Verification items for the finished model (mm, model axes). Give positions to 0.01 mm unless a question says otherwise; leave off trailing zeros. Loops run counter-clockwise (first coordinate to the right, second up) from the corner with the lowest first, then second, coordinate; pieces in that order, holes last. Notation, with made-up numbers: (33, -39) -> (78, -39) arc R12 cw to (78, -28) -> close; hole circle Ø9 at (-40, 40.5). An arc over 180 degrees is marked (long way). Answer in a Markdown table with one row per item. Add a question column.
Q1. Section check B-B on z = 18. Enter the section's corners in (x, y).
Q2. Section check C-C on x = -34.5. Enter the section's corners in (y, z).
Q3. Section check D-D on y = 0.95. Give the number of separate pieces and of enclosed holes in the cut face, and give its area (3 significant figures).
Q4. Section check A-A on x = -16. Enter the section's corners in (y, z).
Q5. Gauge pin test, flat ends, axial feed: P1, Ø0.6, axis at y = 1, z = -34.5, coming from the +X side; P2, Ø0.6, axis at y = 1, z = -34, coming from the +X side. Record the tip position at first contact, or that the pin passes through.
Q6. Material ranges on probe 1 along Z at (x, y) = (-21, 1.85); probe 2 along X at (y, z) = (0.95, -16); probe 3 along Z at (x, y) = (4, 0.3), recorded low to high.
```python
from build123d import *

# Parameters (mm, degrees)
SKETCH1_R           = 1.375
BOSS_EXTRUDE1_DEPTH = 3.1


with BuildPart() as part:
    # Sketch1 → Boss-Extrude1 (new body)
    with BuildSketch(Plane(origin=(0, 0, 0), x_dir=(1, 0, 0), z_dir=(0, 1, 0))):
        with BuildLine():
            Line((-39.71074184, 45.601377345), (28.739257907, 45.601389398))
            ThreePointArc((28.739257907, 45.601389398), (44.917862085, 38.899993272), (51.619259514, 22.721389634))
            Line((51.619259514, 22.721389634), (51.619259514, -33.910586665))
            ThreePointArc((51.619259514, -33.910586665), (48.176660713, -41.25083682), (40.639819253, -44.238608506))
            Line((40.639819253, -44.238608506), (-39.71072563, -44.238622655))
            ThreePointArc((-39.71072563, -44.238622655), (-47.488919901, -41.016788494), (-50.710740093, -33.238588436))
            Line((-50.710740093, -33.238588436), (-50.710740093, 34.601411853))
            ThreePointArc((-50.710740093, 34.601411853), (-47.48890491, 42.379565328), (-39.71074184, 45.601377345))
        make_face()
        with Locations(Location((-45.367589881, 40.25824398, 0), (0, 0, 90))):
            Circle(SKETCH1_R, mode=Mode.SUBTRACT)
        with Locations(Location((-45.367595522, -38.895467925, 0), (0, 0, 90))):
            Circle(SKETCH1_R, mode=Mode.SUBTRACT)
        with Locations(Location((46.094055761, -39.090799779, 0), (0, 0, 90))):
            Circle(SKETCH1_R, mode=Mode.SUBTRACT)
        with Locations(Location((42.796541827, 36.778672843, 0), (0, 0, 90))):
            Circle(SKETCH1_R, mode=Mode.SUBTRACT)
        with BuildLine():
            Line((36.619259514, -24.238609214), (36.619259514, 25.60137805))
            ThreePointArc((36.619259514, 25.60137805), (35.15479342, 29.136911955), (31.619259514, 30.60137805))
            Line((31.619259514, 30.60137805), (-30.710740093, 30.60137805))
            ThreePointArc((-30.710740093, 30.60137805), (-34.246273999, 29.136911955), (-35.710740093, 25.60137805))
            Line((-35.710740093, 25.60137805), (-35.710740093, -24.238609214))
            ThreePointArc((-35.710740093, -24.238609214), (-34.246273999, -27.77414312), (-30.710740093, -29.238609214))
            Line((-30.710740093, -29.238609214), (31.619259514, -29.238609214))
            ThreePointArc((31.619259514, -29.238609214), (35.15479342, -27.77414312), (36.619259514, -24.238609214))
        make_face(mode=Mode.SUBTRACT)
        with BuildLine():
            Line((4.454259711, 35.60137805), (30.619259514, 35.60137805))
            ThreePointArc((30.619259514, 35.60137805), (31.326366295, 35.308484831), (31.619259514, 34.60137805))
            Line((31.619259514, 34.60137805), (31.619259514, 33.50137805))
            ThreePointArc((31.619259514, 33.50137805), (31.326366295, 32.794271268), (30.619259514, 32.50137805))
            Line((30.619259514, 32.50137805), (4.454259711, 32.50137805))
            ThreePointArc((4.454259711, 32.50137805), (3.747152929, 32.794271268), (3.454259711, 33.50137805))
            Line((3.454259711, 33.50137805), (3.454259711, 34.60137805))
            ThreePointArc((3.454259711, 34.60137805), (3.747152929, 35.308484831), (4.454259711, 35.60137805))
        make_face(mode=Mode.SUBTRACT)
        with BuildLine():
            Line((-29.710740093, 35.60137805), (-3.545740289, 35.60137805))
            ThreePointArc((-3.545740289, 35.60137805), (-2.838633508, 35.308484831), (-2.545740289, 34.60137805))
            Line((-2.545740289, 34.60137805), (-2.545740289, 33.50137805))
            ThreePointArc((-2.545740289, 33.50137805), (-2.838633508, 32.794271268), (-3.545740289, 32.50137805))
            Line((-3.545740289, 32.50137805), (-29.710740093, 32.50137805))
            ThreePointArc((-29.710740093, 32.50137805), (-30.417846874, 32.794271268), (-30.710740093, 33.50137805))
            Line((-30.710740093, 33.50137805), (-30.710740093, 34.60137805))
            ThreePointArc((-30.710740093, 34.60137805), (-30.417846874, 35.308484831), (-29.710740093, 35.60137805))
        make_face(mode=Mode.SUBTRACT)
    extrude(amount=BOSS_EXTRUDE1_DEPTH)


solid = part.part
```
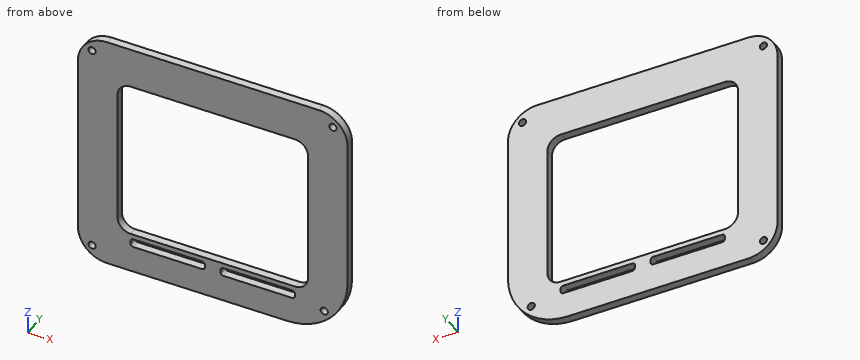
Taken from the geometry:
| question | item | result |
|---|---|---|
| 1 | outline | (-50.71, 0) -> (-35.71, 0) -> (-35.71, 3.1) -> (-50.71, 3.1) -> close; (36.62, 0) -> (51.62, 0) -> (51.62, 3.1) -> (36.62, 3.1) -> close |
| 2 | outline | (0, -45.6) -> (3.1, -45.6) -> (3.1, -28.86) -> (0, -28.86) -> close; (0, 27.5) -> (3.1, 27.5) -> (3.1, 44.24) -> (0, 44.24) -> close |
| 3 | separate pieces | 1 |
| 3 | enclosed holes | 7 |
| 3 | area | 4,500 mm² |
| 4 | outline | (0, -45.6) -> (3.1, -45.6) -> (3.1, -35.6) -> (0, -35.6) -> close; (0, -32.5) -> (3.1, -32.5) -> (3.1, -30.6) -> (0, -30.6) -> close; (0, 29.24) -> (3.1, 29.24) -> (3.1, 44.24) -> (0, 44.24) -> close |
| 5 | P1 | stops at x = 48.53 |
| 5 | P2 | stops at x = 48.81 |
| 6 | probe 1 | z = -45.6 to -35.6, -32.5 to -30.6, 29.24 to 44.24 |
| 6 | probe 2 | x = -50.71 to -35.71, 36.62 to 51.62 |
| 6 | probe 3 | z = -45.6 to -35.49, -32.61 to -30.6, 29.24 to 44.24 |
